Verification items for the finished model (mm, model axes). A direction names the side the tool comes from. Coordinates: 2 decimals unless noted, no trailing zeros. Write each loop counter-clockwise with the first axis right and the second up, starting at its lowest first coordinate (ties: lowest second). Pieces come first, ordered by that corner, then holes. Notation, with made-up numbers: (60.5, -19.75) -> (78.5, -19.75) arc R6 ccw to (78.5, -9.75) -> close; hole circle Ø6 at (-5, -8.5). An arc over 180 degrees is marked (long way). Use CSV: the item, a comma, the result in double quotes.
Autodesk Inventor part; units mm, degrees
ref_plane "Work Plane1" through (0, -1.25, 0) normal (1, 0, 0) x (0, 0, 1)
ref_plane "YZ Plane" through (0, 0, 0) normal (1, 0, 0) x (0, 1, 0)
ref_plane "XZ Plane" through (0, 0, 0) normal (0, 1, 0) x (-1, 0, 0)
sketch "草图1" plane through (0, 0, 0) normal (0, 0, 1) x (1, 0, 0)
  arc A0 (1.5, -19.4383) -> (-1.5, -19.4383) centre (0, -1.25) ccw
  line L0 (0, 47.3657) -> (0, -51.0943)
  line L1 (-46.62, 0) -> (46.62, 0)
  line L2 (-1.5, -19.4383) -> (-1.5, -25.4883)
  line L3 (-1.5, -6.5402) -> (-1.5, -13.29) construction
  line L4 (-2.7947, 22) -> (3.6722, 22) construction
  arc A1 (10.5969, -19.2797) -> (-10.5969, -19.2797) centre (0, 0) ccw
  arc A2 (-9.197, -23.7257) -> (-1.5, -25.4883) centre (0, -1.25) ccw
  arc A3 (-9.5, -23.3498) -> (-9.197, -23.7257) centre (-9.0076, -23.263) ccw
  arc A4 (-10.0938, -19.9824) -> (-10.5969, -19.2797) centre (-11.0786, -20.156) ccw
  line L5 (1.5, -19.4383) -> (1.5, -25.4883)
  line L6 (1.5, -6.5402) -> (1.5, -13.29) construction
  arc A5 (1.5, -25.4883) -> (9.197, -23.7257) centre (0, -1.25) ccw
  arc A6 (9.197, -23.7257) -> (9.5, -23.3498) centre (9.0076, -23.263) ccw
  circle A7 centre (-5.5, -21.8277) radius 1.25
  circle A8 centre (5.5, -21.8277) radius 1.25
  line L7 (-10.0938, -19.9824) -> (-9.5, -23.3498)
  arc A9 (10.5969, -19.2797) -> (10.0938, -19.9824) centre (11.0786, -20.156) ccw
  line L8 (9.5, -23.3498) -> (10.0938, -19.9824)
  arc A10 (-2.7484, -22.3719) -> (3.183, -22.3108) centre (0, -1.25) ccw construction
  dimension "d0" = 36.5
  dimension "d1" = 6.05
  dimension "d6" = 1.5
  dimension "d8" = 1.25
  dimension "d9" = 0.5
  dimension "d10" = 1
  dimension "d12" = 2.5
  dimension "d13" = 2.5
  dimension "d43" = 10
  dimension "d44" = 21.3
  dimension "d45" = 11
  dimension "d46" = 19
  dimension "d47" = 5
extrude "轴承体" add sketch "草图1" along normal blind 1.5 contours A0 L1 A1 A9 L8 A6 A5 L5 | A0 L0 A1 L1 | A0 L1 A1 L0 | A0 L2 A2 A3 L7 A4 A1 L1
ref_plane "Work Plane1" through (0, -1.25, 0) normal (1, 0, 0) x (0, 0, 1)
equation "\"d0\" = ND"
equation "\"d1\" = SRB2"
equation "\"d6\" = 0.5 * B1"
equation "\"d8\" = C1"
equation "\"d9\" = R3"
equation "\"d10\" = R2"
equation "\"d12\" = SD5"
equation "\"d13\" = SD5"
equation "\"d44\" = R1"
equation "\"d45\" = B2"
equation "\"d46\" = L"
equation "\"d47\" = SRB1"
equation "\"d2\" = SD"
equation "\"SD\" = 1.5"
equation "\"SRB1\" = 5"
equation "\"ND\" = 36.5"
equation "\"SRB2\" = 6.05"
equation "\"SD5\" = 2.5"
equation "\"B1\" = 3"
equation "\"R2\" = 1"
equation "\"R3\" = 0.5"
equation "\"B2\" = 11"
equation "\"R1\" = 21.3"
equation "\"C1\" = 1.25"
equation "\"SD3\" = 36.5"
equation "\"WDMAX\" = 42"
equation "\"H1\" = 0"
properties part number "弹性挡圈GB 894.1-86 - 40" material "钢，软"
1) Mould release check, pull along X, two halves, no side actions. Record for faces 1 (the flat face through (-9.8, -21.64, 0.74)), 2 (the cylindrical face through (5.337, -23.067, 0.74)), 3 (the flat face through (0, 18, 0)), 4 (the cylindrical face through (-5.663, -23.067, 0.74)): released by +X, released by -X, zero draft, split by the parting line, or undercut.
Return value:
face 1,"released by -X"
face 2,"undercut"
face 3,"zero draft"
face 4,"undercut"
2) Cross-section at C-C (z = 1.1). Record the boundary of the cut face in (x, y).
Return value:
outline,"(-10.6, -19.28) arc R1 cw to (-10.09, -19.98) -> (-9.5, -23.35) arc R0.5 ccw to (-9.2, -23.73) arc R24.29 ccw to (-1.5, -25.49) -> (-1.5, -19.44) arc R18.25 cw (long way) to (1.5, -19.44) -> (1.5, -25.49) arc R24.28 ccw to (9.2, -23.73) arc R0.5 ccw to (9.5, -23.35) -> (10.09, -19.98) arc R1 cw to (10.6, -19.28) arc R22 ccw (long way) to start; hole circle Ø2.5 at (-5.5, -21.83); hole circle Ø2.5 at (5.5, -21.83)"
3) Cross-section at B-B (y = -6.5). Record the boundary of the cut face in (x, z).
Return value:
outline,"(-21.02, 0) -> (-17.48, 0) -> (-17.48, 1.5) -> (-21.02, 1.5) -> close; (17.48, 0) -> (21.02, 0) -> (21.02, 1.5) -> (17.48, 1.5) -> close"
4) Gauge pin test, flat end, axial feed: pin 1 (1.5 mm diameter, centred on x = -5.5, y = -21.83, fed in from +Z). Record the tip position at first contact, or that the pin passes through.
Return value:
pin 1,"through"
5) Cross-section at A-A (x = 5.5). Record the boundary of the cut face in (y, z), plus the area to 3 significant figures.
Return value:
outline,"(-24.9, 0) -> (-23.08, 0) -> (-23.08, 1.5) -> (-24.9, 1.5) -> close; (-20.58, 0) -> (-18.65, 0) -> (-18.65, 1.5) -> (-20.58, 1.5) -> close; (16.15, 0) -> (21.3, 0) -> (21.3, 1.5) -> (16.15, 1.5) -> close"
area,"13.4 mm2"
6) Scan lines: L1, parallel to Y at x = 5.5, z = 0.5; L2, parallel to Y at x = 0, z = 1.1; L3, parallel to X at y = -11.5, z = 0.95. Record each from-to range of solid material in increasing order.
Return value:
L1,"-24.9 to -23.08, -20.58 to -18.65, 16.15 to 21.3"
L2,"17 to 22"
L3,"-18.76 to -15.1, 15.1 to 18.76"
7) Set-up check for faces 5 (the flat face through (9.793, -21.69, 0.74)), 6 (the flat face through (1.5, -22, 1)): record each of +Z, -Z, +X, -X, +Y, -Y from which the full face is reachable in a straight line by a thin tool's end or side.
Return value:
face 5,"+Z, -Z, +X, -Y"
face 6,"+Z, -Z, -Y"
8) Cross-section at D-D (x = -3). Record the boundary of the cut face in (y, z).
Return value:
outline,"(-25.35, 0) -> (-19.25, 0) -> (-19.25, 1.5) -> (-25.35, 1.5) -> close; (16.75, 0) -> (21.79, 0) -> (21.79, 1.5) -> (16.75, 1.5) -> close"
